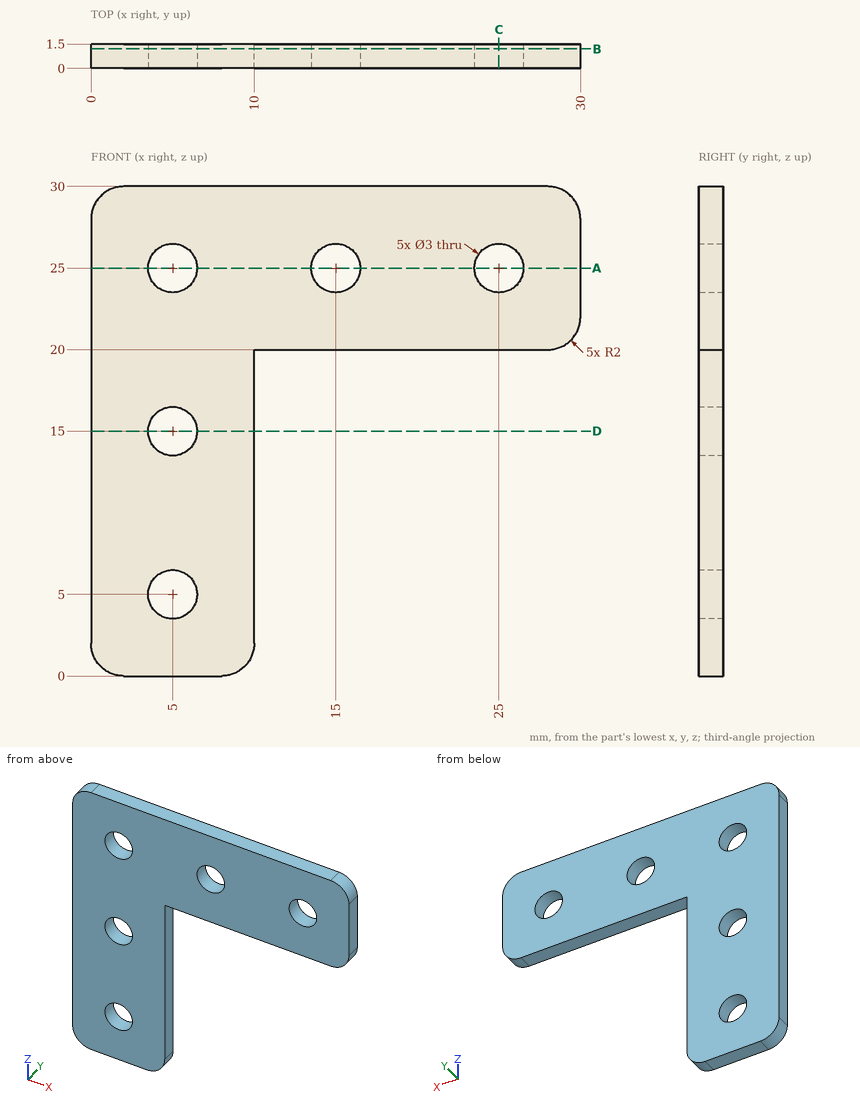
Design review of the part shown in the three views and the two pictorial views. Dimensions are in mm from the part's minimum x, y and z. Coordinates: 2 decimals unless noted, no trailing zeros. Order: outer loops, then holes, each group sorted by start corner. A loop starts at its lowest first (then second) coordinate and runs counter-clockwise, first axis right, second up. Notation, with made-up numbers: (-23.5, 63.5) - (12.5, 63.5) arc R27 cw to (12.5, 96.5) - close; hole circle Ø9 at (-29, 89). An arc over 180 degrees is marked (long way). Answer as CSV lines item,"result". Start each with the question number.
1) Add section D-D (z = 15). State the section outline as (x, y) points, then the cut area to 3 significant figures.
2) Add section A-A (z = 25). State the section outline as (x, y) points, then the cut area to 3 significant figures.
3) Add section B-B (y = 1.2). State the section outline as (x, z) points, then the cut area to 3 significant figures.
4) Add section C-C (x = 25). State the section outline as (y, z) points.
5) Insertion check: P1, Ø0.8, axis at x = 19.5, y = 1, coming from the -Z side. The pin has a flat end and moves straight along its axis. Give the tip position at first contact, or say it passes through.
6) To check wall thickness, follow line 1 along X through (y, z) = (0.55, 25); line 2 along X through (y, z) = (0.35, 5); line 3 along Z through (x, y) = (11.5, 0.1). State the ranges of each line that lie inside material, in increasing order. Write a range as [from, to].
Result:
1,outline,"(0, 0) - (3.5, 0) - (3.5, 1.5) - (0, 1.5) - close; (6.5, 0) - (10, 0) - (10, 1.5) - (6.5, 1.5) - close"
1,area,"10.5 mm^2"
2,outline,"(0, 0) - (3.5, 0) - (3.5, 1.5) - (0, 1.5) - close; (6.5, 0) - (13.5, 0) - (13.5, 1.5) - (6.5, 1.5) - close; (16.5, 0) - (23.5, 0) - (23.5, 1.5) - (16.5, 1.5) - close; (26.5, 0) - (30, 0) - (30, 1.5) - (26.5, 1.5) - close"
2,area,"31.5 mm^2"
3,outline,"(0, 2) arc R2 ccw to (2, 0) - (8, 0) arc R2 ccw to (10, 2) - (10, 20) - (28, 20) arc R2 ccw to (30, 22) - (30, 28) arc R2 ccw to (28, 30) - (2, 30) arc R2 ccw to (0, 28) - close; hole circle Ø3 at (5, 5); hole circle Ø3 at (5, 15); hole circle Ø3 at (5, 25); hole circle Ø3 at (15, 25); hole circle Ø3 at (25, 25)"
3,area,"460 mm^2"
4,outline,"(0, 20) - (1.5, 20) - (1.5, 23.5) - (0, 23.5) - close; (0, 26.5) - (1.5, 26.5) - (1.5, 30) - (0, 30) - close"
5,P1,"z = 20"
6,line 1,"[0, 3.5], [6.5, 13.5], [16.5, 23.5], [26.5, 30]"
6,line 2,"[0, 3.5], [6.5, 10]"
6,line 3,"[20, 30]"
